```python
from build123d import *

# Parameters (mm, degrees)
F0_R     = 37.5
F0_R_2   = 2
F1_DEPTH = 2
F2_R     = 4
F3_DEPTH = 1


with BuildPart() as f1:
    # F0 (on Top) → F1 (new body)
    with BuildSketch(Plane.XY):
        Circle(F0_R)
        with Locations((-23, -23)):
            Circle(F0_R_2, mode=Mode.SUBTRACT)
        with Locations((23, -23)):
            Circle(F0_R_2, mode=Mode.SUBTRACT)
        with Locations((-23, 23)):
            Circle(F0_R_2, mode=Mode.SUBTRACT)
        with Locations((23, 23)):
            Circle(F0_R_2, mode=Mode.SUBTRACT)
    extrude(amount=F1_DEPTH)

    # F2 (on face) → F3 (cut)
    with BuildSketch(Plane.XY.offset(2)):
        with Locations((-23, 23)):
            Circle(F2_R)
        with Locations((23, 23)):
            Circle(F2_R)
        with Locations((-23, -23)):
            Circle(F2_R)
        with Locations((23, -23)):
            Circle(F2_R)
    extrude(amount=-F3_DEPTH, mode=Mode.SUBTRACT)


solid = f1.part
```
Source: CAD feature listing. Evaluate the final solid. Frame: model axes, mm. A direction names the side the tool comes from. Give positions to 0.01 mm unless a question says otherwise; leave off trailing zeros. Loops run counter-clockwise (first coordinate to the right, second up) from the corner with the lowest first, then second, coordinate; pieces in that order, holes last. Notation, with made-up numbers: (-25, -19.5) - (27, -19.5) arc R17 cw to (27, -6.5) - close; hole circle Ø7 at (7.5, 86). An arc over 180 degrees is marked (long way). Use CSV: the item, a comma, the result in double quotes.
1) Cut plane C-C (y = -26). Output: boundary loops of the cut face in (x, z).
Worked out:
outline,"(-27.02, 0) - (27.02, 0) - (27.02, 2) - (25.65, 2) - (25.65, 1) - (20.35, 1) - (20.35, 2) - (-20.35, 2) - (-20.35, 1) - (-25.65, 1) - (-25.65, 2) - (-27.02, 2) - close"
2) Cut plane D-D (x = 13). Output: boundary loops of the cut face in (y, z).
Worked out:
outline,"(-35.17, 0) - (35.17, 0) - (35.17, 2) - (-35.17, 2) - close"
3) Mould query, pull axis X, two halves, no side actions, for faces 1 (the cylindrical face through (-4.88, 37.18, 0.99)), 2 (the cylindrical face through (21.526, -21.648, 0.493)), 3 (the flat face through (-1, 1, 2)). Classes: +X half, -X half, draft (parallel to the pull), parting line (faces both ways), or undercut.
Worked out:
face 1,"parting line"
face 2,"undercut"
face 3,"draft"
4) Pin query (flat end, axial travel): P1, Ø4, axis at x = 24.5, y = -23, coming from the +Z side. Return the tip coordinate at first contact, or that it passes through.
Worked out:
P1,"stops at z = 1"
5) Cut plane A-A (z = 1.6). Output: boundary loops of the cut face in (x, y), and give its area (3 significant figures).
Worked out:
outline,"circle Ø75 at (0, 0); hole circle Ø8 at (-23, -23); hole circle Ø8 at (-23, 23); hole circle Ø8 at (23, -23); hole circle Ø8 at (23, 23)"
area,"4,220 mm^2"
6) Set-up query: faces 4 (the flat face through (-22, -21, 1)), 5 (the cylindrical face through (-24.474, -21.648, 0.493)). Return all of +Z, -Z, +X, -X, +Y, -Y with unobstructed straight access to the full face (end or side cutting, diameter ignored); none if empty.
Worked out:
face 4,"+Z"
face 5,"+Z, -Z"
7) Cut plane B-B (x = -24). Output: boundary loops of the cut face in (y, z), and give its area (3 significant figures).
Worked out:
outline,"(-28.81, 0) - (-24.73, 0) - (-24.73, 1) - (-26.87, 1) - (-26.87, 2) - (-28.81, 2) - close; (-21.27, 0) - (21.27, 0) - (21.27, 1) - (19.13, 1) - (19.13, 2) - (-19.13, 2) - (-19.13, 1) - (-21.27, 1) - close; (24.73, 0) - (28.81, 0) - (28.81, 2) - (26.87, 2) - (26.87, 1) - (24.73, 1) - close"
area,"92.8 mm^2"
8) Line query: line 1 (X direction, y = 23, z = 0.85); line 2 (Y direction, x = 23, z = 1.7). Output: solid intervals per line, ascending.
Worked out:
line 1,"x = -29.62 to -25, -21 to 21, 25 to 29.62"
line 2,"y = -29.62 to -27, -19 to 19, 27 to 29.62"
